Design review of the part built by this model. Coordinates are the model's own, in mm. Round coordinates to 2 decimals unless told otherwise and drop trailing zeros. Loops run counter-clockwise (first coordinate to the right, second up) from the corner with the lowest first, then second, coordinate; pieces in that order, holes last. Notation, with made-up numbers: (87, -34) - (139, -34) arc R13 cw to (139, -11) - close; hole circle Ø8 at (-22.5, 40). An arc over 180 degrees is marked (long way). Use one line per item in the form item = value. Start each with the question number.
(1) For pin 1 (1.5 mm diameter, centred on y = 2.5, z = -0.5, fed in from +X); pin 2 (3.5 mm diameter, centred on x = -32.85, z = -12.39, fed in from -Y), all flat-tipped, find the tip position at first contact; note any pin that passes through.
(2) We need section A-A, the plane x = -68. Write out the cut boundary in (y, z), then the cut area to 3 significant figures.
(3) The part is to be moulded in two halves that separate along X. For faces 1 (the cylindrical face through (-30.32, 0.07, 14)), 2 (the cylindrical face through (1.246, -1.978, 2.579)), say which applies: released by +X, released by -X, zero draft, split by the parting line, or undercut.
(4) We need section B-B, the plane z = 0. Write out the cut boundary in (x, y).
(5) We need section C-C, the plane x = -8. Write out the cut boundary in (y, z), then the cut area to 3 significant figures.
(6) Wall thickness on probe 1 along Z at (x, y) = (-68, 1.25); probe 2 along Y at (x, z) = (-12.5, -3); probe 3 along Z at (x, y) = (50, -2.75): over which ranges is each line inside the solid? List them lowest first. Write a range as [from, to].
from build123d import *

# Parameters (mm, degrees)
SKETCH1_W           = 180
SKETCH1_H           = 35
BOSS_EXTRUDE1_DEPTH = 5
SKETCH3_R           = 3.25
CUT_EXTRUDE1_DEPTH  = 181.917799014
CHAMFER1_SIZE       = 1
CHAMFER2_SIZE       = 1
SKETCH5_R           = 1.5
CUT_EXTRUDE2_DEPTH  = 10
SKETCH18_R          = 1.5
CUT_EXTRUDE3_DEPTH  = 36
SKETCH19_R          = 3
CUT_EXTRUDE4_DEPTH  = 10


with BuildPart() as part:
    # Sketch1 → Boss-Extrude1 (new, symmetric)
    with BuildSketch(Plane(origin=(0, 0, 0), x_dir=(1, 0, 0), z_dir=(0, 1, 0))):
        Rectangle(SKETCH1_W, SKETCH1_H)
    extrude(amount=BOSS_EXTRUDE1_DEPTH, both=True)

    # Sketch3 → Cut-Extrude1 (cut, through all)
    with BuildSketch(Plane(origin=(90, 0, 0), x_dir=(0, 0, -1), z_dir=(1, 0, 0))):
        Circle(SKETCH3_R)
    extrude(amount=-CUT_EXTRUDE1_DEPTH, mode=Mode.SUBTRACT)

    # Chamfer1
    chamfer1_edges = [part.edges().sort_by_distance(p)[0] for p in [
        (90, 0, 3.25),
    ]]
    chamfer(chamfer1_edges, length=CHAMFER1_SIZE)

    # Chamfer2
    chamfer2_edges = [part.edges().sort_by_distance(p)[0] for p in [
        (-90, 0, 3.25),
    ]]
    chamfer(chamfer2_edges, length=CHAMFER2_SIZE)

    # Sketch5 → Cut-Extrude2 (cut)
    with BuildSketch(Plane(origin=(0, 5, 0), x_dir=(1, 0, 0), z_dir=(0, 1, 0))):
        with Locations(Location((-68, -11.2, 0), (0, 0, 270))):
            Circle(SKETCH5_R)
        with Locations(Location((-68, 11.2, 0), (0, 0, 270))):
            Circle(SKETCH5_R)
        with Locations(Location((24, 11.2, 0), (0, 0, 270))):
            Circle(SKETCH5_R)
        with Locations(Location((24, -11.2, 0), (0, 0, 270))):
            Circle(SKETCH5_R)
    extrude(amount=-CUT_EXTRUDE2_DEPTH, mode=Mode.SUBTRACT)

    # Sketch18 → Cut-Extrude3 (cut)
    with BuildSketch(Plane(origin=(0, 5, 0), x_dir=(1, 0, 0), z_dir=(0, 1, 0))):
        with Locations(Location((-75.552597146, 13, 0), (0, 0, 270))):
            Circle(SKETCH18_R)
        with Locations(Location((-75.552597146, -13, 0), (0, 0, 270))):
            Circle(SKETCH18_R)
        with Locations(Location((7.447402854, -13, 0), (0, 0, 270))):
            Circle(SKETCH18_R)
        with Locations(Location((7.447402854, 13, 0), (0, 0, 270))):
            Circle(SKETCH18_R)
    extrude(amount=-CUT_EXTRUDE3_DEPTH, mode=Mode.SUBTRACT)

    # Sketch19 → Cut-Extrude4 (cut)
    with BuildSketch(Plane(origin=(0, 5, 0), x_dir=(1, 0, 0), z_dir=(0, 1, 0))):
        with Locations(Location((-84.632352591, 12.390150385, 0), (0, 0, 270))):
            Circle(SKETCH19_R)
        with Locations(Location((-84.632352591, -12.390150385, 0), (0, 0, 270))):
            Circle(SKETCH19_R)
        with Locations(Location((83.204027378, 12.390150385, 0), (0, 0, 270))):
            Circle(SKETCH19_R)
        with Locations(Location((83.204027378, -12.390150385, 0), (0, 0, 270))):
            Circle(SKETCH19_R)
        with Locations(Location((42.676245092, -12.390150385, 0), (0, 0, 270))):
            Circle(SKETCH19_R)
        with Locations(Location((42.676245092, 12.390150385, 0), (0, 0, 270))):
            Circle(SKETCH19_R)
        with Locations(Location((-32.852727664, -12.390150385, 0), (0, 0, 270))):
            Circle(SKETCH19_R)
        with Locations(Location((-32.852727664, 12.390150385, 0), (0, 0, 270))):
            Circle(SKETCH19_R)
    extrude(amount=-CUT_EXTRUDE4_DEPTH, mode=Mode.SUBTRACT)


solid = part.part
Data:
q1.pin_1 = 89.05
q1.pin_2 = through
q2.outline = (-5, -17.5) - (5, -17.5) - (5, -12.7) - (-5, -12.7) - close; (-5, -9.7) - (5, -9.7) - (5, 9.7) - (-5, 9.7) - close; (-5, 12.7) - (5, 12.7) - (5, 17.5) - (-5, 17.5) - close; hole circle Ø6.5 at (0, 0)
q2.area = 257 mm^2
q3.face_1 = undercut
q3.face_2 = zero draft
q4.outline = (-90, -5) - (90, -5) - (90, -4.25) - (89, -3.25) - (-89, -3.25) - (-90, -4.25) - close; (-90, 4.25) - (-89, 3.25) - (89, 3.25) - (90, 4.25) - (90, 5) - (-90, 5) - close
q5.outline = (-5, -17.5) - (5, -17.5) - (5, 17.5) - (-5, 17.5) - close; hole circle Ø6.5 at (0, 0)
q5.area = 317 mm^2
q6.probe_1 = [-17.5, -12.7], [-9.7, -3], [3, 9.7], [12.7, 17.5]
q6.probe_2 = [-5, -1.25], [1.25, 5]
q6.probe_3 = [-17.5, -1.73], [1.73, 17.5]
